For this review, take the finished solid that the model builds, in its own axes (mm). A direction names the side the tool comes from. Round coordinates to 2 decimals unless told otherwise and drop trailing zeros. Order: outer loops, then holes, each group sorted by start corner. A loop starts at its lowest first (then second) coordinate and runs counter-clockwise, first axis right, second up. Notation, with made-up numbers: (72.5, 11) -> (119.5, 11) arc R20 ccw to (119.5, 45) -> close; hole circle Ø5 at (72.5, 73.25). An arc over 180 degrees is marked (long way). Answer in a Markdown table with one row per item.
Autodesk Inventor part; units mm, degrees
ref_plane "YZ Plane" through (0, 0, 0) normal (1, 0, 0) x (0, 1, 0)
ref_plane "XZ Plane" through (0, 0, 0) normal (0, 1, 0) x (-1, 0, 0)
ref_plane "XY Plane" through (0, 0, 0) normal (0, 0, 1) x (1, 0, 0)
sketch "スケッチ1" plane through (0, 0, 0) normal (0, 0, 1) x (1, 0, 0)
  arc A0 (0.7632, 11.9121) -> (-1.0179, 11.893) centre (0, 0) ccw construction
  arc A1 (0.4062, 11.3607) -> (-0.4062, 11.3607) centre (0, 0) ccw
  arc A2 (9.3048, 1.5803) -> (-9.0567, 2.6555) centre (0, 0) ccw construction
  arc A3 (0.8923, 10.7753) -> (1.9623, 9.2318) centre (2.2471, 10.5718) ccw
  line L0 (1.9623, 9.2318) -> (0, 0)
  arc A4 (-1.9623, 9.2318) -> (-0.8923, 10.7753) centre (-2.2471, 10.5718) ccw
  line L1 (-1.9623, 9.2318) -> (0, 0)
  arc A5 (-0.4062, 11.3607) -> (-0.8923, 10.7753) centre (-0.388, 10.8511) ccw
  arc A6 (0.8923, 10.7753) -> (0.4062, 11.3607) centre (0.388, 10.8511) ccw
  line L2 (0, 0) -> (0, 2.9942) construction
  dimension "d0" = 11.9365
  dimension "d1" = 11.368
  dimension "d2" = 1.93
  dimension "d3" = 0.51
  dimension "d4" = 1.37
  dimension "d5" = 1.37
  dimension "d6" = 24
  dimension "d7" = 12
extrude "押し出し1" add sketch "スケッチ1" along normal blind 5
pattern_circular "円形状パターン1" count 15 over 360 about axis through (0, 0, 0) along (0, 0, 1) of "押し出し1"
sketch "スケッチ2" plane through (0, 0, 5) normal (0, 0, 1) x (1, 0, 0)
  circle A0 centre (0, 0) radius 14
  dimension "d13" = 28
extrude "押し出し2" add sketch "スケッチ2" along normal blind 1
sketch "スケッチ3" plane through (0, 0, 0) normal (0, 0, -1) x (-1, 0, 0)
  circle A0 centre (0, 0) radius 4
  circle A1 centre (0, 7) radius 1.6
  circle A2 centre (-7, 0) radius 1.6
  circle A3 centre (7, 0) radius 1.6
  dimension "d16" = 8
  dimension "d18" = 3.2
  dimension "d19" = 7
  dimension "d20" = 3.2
  dimension "d21" = 3.2
  dimension "d22" = 7
  dimension "d23" = 7
extrude "押し出し3" cut sketch "スケッチ3" against normal through all
properties part number "プーリ_歯数15" material "アセタール樹脂、白"
Q1. Take a section at A-A, the plane y = -3.5. Write out the cut boundary in (x, z), then the cut area to 3 significant figures.
Answer key:
| item | result |
|---|---|
| outline | (-13.56, 5) -> (-8.92, 5) -> (-8.92, 0) -> (-1.94, 0) -> (-1.94, 6) -> (-13.56, 6) -> close; (1.94, 0) -> (8.92, 0) -> (8.92, 5) -> (13.56, 5) -> (13.56, 6) -> (1.94, 6) -> close |
| area | 93.1 mm^2 |
Q2. Tool access review of faces 4 (the face through (-5.004, 8.503, 2.465)), 5 (the face through (-0.95, -9.82, 2.46)), 6 (the face through (-9.667, 1.971, 2.465)): name each direction out of +Z, -Z, +X, -X, +Y, -Y from which nothing blocks a thin tool from reaching the whole face with its end or side.
Answer key:
| item | result |
|---|---|
| face 4 | -Z |
| face 5 | -Z, -Y |
| face 6 | -Z, -X |
Q3. To check wall thickness, follow probe 1 along Y at (x, z) = (0, 4.15); probe 2 along X at (y, z) = (-9.75, 1.55); probe 3 along Y at (x, z) = (-7, 3.5). State the ranges of each line that lie inside material, in increasing order.
Answer key:
| item | result |
|---|---|
| probe 1 | y = -9.44 to -4, 4 to 5.4, 8.6 to 11.37 |
| probe 2 | x = -3.03 to -0.87, 0.87 to 3.03 |
| probe 3 | y = -8.96 to -8.13, -6.33 to -1.6, 1.6 to 7.54 |
Q4. Take a section at C-C, the plane z = 4.2. Give the number of separate pieces and of enclosed holes in the cut face, then the cut area to 3 significant figures.
Answer key:
| item | result |
|---|---|
| separate pieces | 1 |
| enclosed holes | 4 |
| area | 263 mm^2 |
Q5. Clearance check with a flat-ended pin moving along its axis: pin 1 Ø3 at (x, z) = (-2.5, 1.5) entering from +Y. State where the tip first meets the part, or that it passes through.
Answer key:
| item | result |
|---|---|
| pin 1 | stops at y = 10.58 |
Q6. Take a section at B-B, the plane y = -6.75. Write out the cut boundary in (x, z), then the cut area to 3 significant figures.
Answer key:
| item | result |
|---|---|
| outline | (-12.27, 5) -> (-6.75, 5) -> (-6.75, 0) -> (6.75, 0) -> (6.75, 5) -> (12.27, 5) -> (12.27, 6) -> (-12.27, 6) -> close |
| area | 92.0 mm^2 |
Q7. The part is to be moulded in two halves that separate along X. For faces 1 (the face through (-11.305, -1.194, 2.465)), 2 (the face through (4.834, -8.576, 2.465)), 3 (the face through (9.65, 1.95, 2.46)), say which applies: +X half, -X half, draft (parallel to the pull), parting line (faces both ways), or undercut.
Answer key:
| item | result |
|---|---|
| face 1 | -X half |
| face 2 | undercut |
| face 3 | +X half |
